Answer from the drawing. Dimensions are ordinates in mm from the lowest x, y and z of the part. A direction names the side the tool comes from. Give positions to 0.01 mm unless a question says otherwise; leave off trailing zeros. Write each loop counter-clockwise with the first axis right and the second up, starting at its lowest first coordinate (ties: lowest second). Pieces come first, ordered by that corner, then holes.
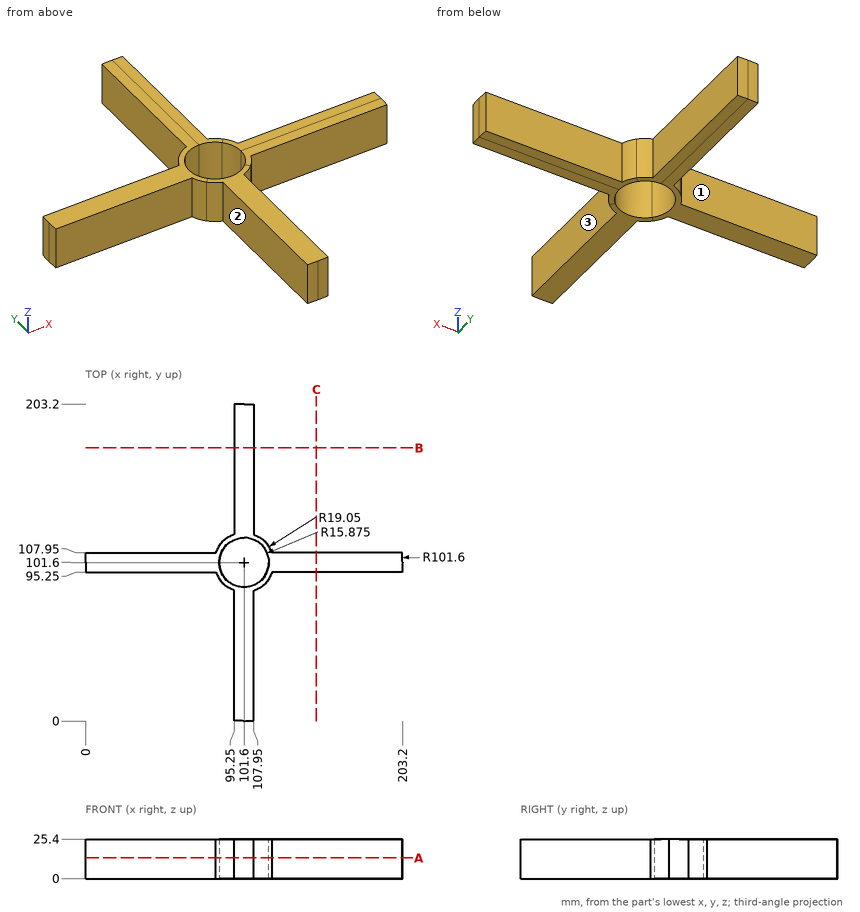
Item 1: Which of the six approach directions +Z, -Z, +X, -X, +Y, -Y give full straight-line access (tool end or side, diameter ignored) to the marked faces 1, 2 and 3?
Conclusion:
face 1: +Z, -Z, -X, +Y
face 2: +Z, -Z, -X, -Y
face 3: +Z, -Z, +X, -Y
Item 2: Consider probe 1 along X at (y, z) = (194.5, 13); probe 2 along X at (y, z) = (103, 6.5). Determine where each line is inside the solid, lowest interval first.
Conclusion:
probe 1: x = 95.25 to 107.95
probe 2: x = 0.01 to 85.79, 117.41 to 203.19
Item 3: A cutting plane is placed at A-A, the plane z = 13.25. Give the vertices of the cut face in (x, y) (3 decimals), plus the area to 3 significant figures.
Conclusion:
outline: (0.199, 95.25) - (83.639, 95.25) arc R19.05 ccw to (95.25, 83.639) - (95.25, 0.199) arc R101.6 ccw to (107.95, 0.199) - (107.95, 83.639) arc R19.05 ccw to (119.561, 95.25) - (203.001, 95.25) arc R101.6 ccw to (203.001, 107.95) - (119.561, 107.95) arc R19.05 ccw to (107.95, 119.561) - (107.95, 203.001) arc R101.6 ccw to (95.25, 203.001) - (95.25, 119.561) arc R19.05 ccw to (83.639, 107.95) - (0.199, 107.95) arc R101.6 ccw to start; hole circle Ø31.75 at (101.6, 101.6)
area: 4,560 mm2
Item 4: A cutting plane is placed at B-B, the plane y = 175. Give the vertices of the cut face in (x, z).
Conclusion:
outline: (95.25, 0) - (107.95, 0) - (107.95, 25.4) - (95.25, 25.4) - close
Item 5: Each of these flat-tipped pins is pushed along its axis until it touches: P1, Ø4, axis at x = 152.5, z = 14.5, coming from the +Y side; P2, Ø1, axis at y = 182, z = 11, coming from the +X side; P3, Ø7.5, axis at y = 157.5, z = 7.5, coming from the -X side. Where does it stop, or does it pass through?
Conclusion:
P1: stops at y = 107.95
P2: stops at x = 107.95
P3: stops at x = 95.25
